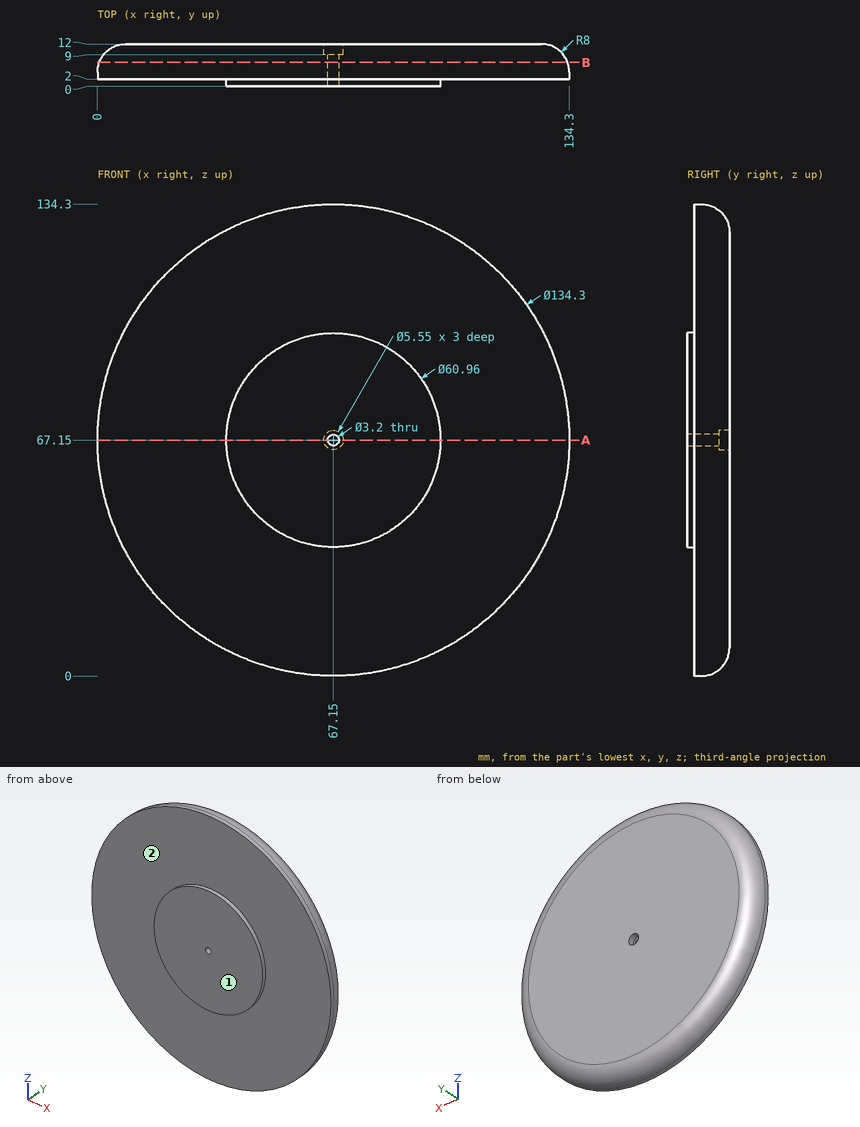
Drawing for the job (mm, zero at the part's lowest x, y, z). A direction names the side the tool comes from. Round coordinates to 2 decimals unless told otherwise and drop trailing zeros. Loops run counter-clockwise (first coordinate to the right, second up) from the corner with the lowest first, then second, coordinate; pieces in that order, holes last. Notation, with made-up numbers: (-31.75, 86.25) -> (4.25, 86.25) arc R15 cw to (4.25, 111.25) -> close; hole circle Ø8 at (29, 1.5). An arc over 180 degrees is marked (long way). Answer in a Markdown table with one row per item.
Item 1: Which spindle directions (+Z, -Z, +X, -X, +Y, -Y) get a long thin tool onto all of the face, cutting with end or side? Do the marked faces 1 and 2. Say none if no direction does.
Answers below:
| item | result |
|---|---|
| face 1 | +Z, -Z, +X, -X, -Y |
| face 2 | -Y |
Item 2: Saw through at A-A (z = 67.15). Write the cut outline in (x, y) (3 decimals).
Answers below:
| item | result |
|---|---|
| outline | (0, 2) -> (36.67, 2) -> (36.67, 0) -> (65.55, 0) -> (65.55, 9) -> (64.375, 9) -> (64.375, 12) -> (8, 12) arc R8 ccw to (0, 4) -> close; (68.75, 0) -> (97.63, 0) -> (97.63, 2) -> (134.3, 2) -> (134.3, 4) arc R8 ccw to (126.3, 12) -> (69.925, 12) -> (69.925, 9) -> (68.75, 9) -> close |
Item 3: Saw through at B-B (y = 6.75). Write the cut outline in (x, z).
Answers below:
| item | result |
|---|---|
| outline | circle Ø133.32 at (67.15, 67.15); hole circle Ø3.2 at (67.15, 67.15) |
Item 4: Drill centre lines: L1, parallel to X at y = 3.5, z = 67.15; L2, parallel to Y at x = 126, z = 71.5; L3, parallel to X at y = 6.25, z = 67.15. Where is each one in solid material? Low to high. Write a range as [from, to].
Answers below:
| item | result |
|---|---|
| L1 | x = [0, 65.55], [68.75, 134.3] |
| L2 | y = [2, 12] |
| L3 | x = [0.32, 65.55], [68.75, 133.98] |
Item 5: Pin check, flat tips, straight feed: pin 1 (6 mm diameter, centred on y = 8, z = 75, fed in from -X); pin 2 (5 mm diameter, centred on y = 1, z = 20.5, fed in from -X); pin 3 (2 mm diameter, centred on x = 16, y = 3.5, fed in from -Z). Stop position of each tip, or through.
Answers below:
| item | result |
|---|---|
| pin 1 | stops at x = 0.43 |
| pin 2 | stops at x = 16.74 |
| pin 3 | stops at z = 22.49 |
